from build123d import *

# Parameters (mm, degrees)
F0_R     = 19.355113
F1_DEPTH = 17.5
F2_R     = 5
F3_R     = 5


with BuildPart() as f1:
    # F0 (on Front) → F1 (new body, symmetric)
    with BuildSketch(Plane.XZ):
        Circle(F0_R)
    extrude(amount=F1_DEPTH, both=True)

    # F2
    f2_edges = [f1.edges().sort_by_distance(p)[0] for p in [
        (-19.355113, -17.5, 0),
    ]]
    fillet(f2_edges, radius=F2_R)

    # F3
    f3_edges = [f1.edges().sort_by_distance(p)[0] for p in [
        (-19.355113, 17.5, 0),
    ]]
    fillet(f3_edges, radius=F3_R)


solid = f1.part
The listing builds one solid part. Answer for the finished solid, in the listing's coordinates (mm). Round coordinates to 2 decimals unless told otherwise and drop trailing zeros. Write each loop counter-clockwise with the first axis right and the second up, starting at its lowest first coordinate (ties: lowest second). Pieces come first, ordered by that corner, then holes. Notation, with made-up numbers: M 2.5,84.25 L 32.5,84.25 A11 ccw 32.5,101.25 Z; hole C -29,-11.75 d2. An arc over 180 degrees is marked long. Write each question's results on one line, items separated by ' | '. Start each with the question number.
Item 1: Flat-ended cylindrical pins translate along their axes: pin 1 Ø1.5 at (x, z) = (13.5, 13.5) entering from +Y; pin 2 Ø6 at (x, y) = (-11, 7) entering from +Z; pin 3 Ø5 at (x, y) = (10, -7) entering from +Z. Find the tip coordinate at first contact, or state that the pin passes through.
Item 2: For a pull along X with two mould halves and no side action, classify faces 1 (the face through (0, -17.5, 0)), 2 (the face through (18.461, -0.175, 5.814)) as pulls with the +X half, pulls with the -X half, needs draft (parallel to the pull), parting line crosses it, or undercut.
Item 3: A cutting plane is placed at C-C on y = 10.5. Write down the section's boundary in (x, z), and give its area (3 significant figures).
Item 4: A cutting plane is placed at B-B on z = 0. Write down the section's boundary in (x, y), and give its area (3 significant figures).
Item 5: A cutting plane is placed at A-A on x = 0. Write down the section's boundary in (y, z).
Item 6: Straight lines are drawn through the part: L1, parallel to Y at x = -11.5, z = 12.5; L2, parallel to Y at x = 14, z = -5; L3, parallel to X at y = -5, z = 11. For each, find the intervals that lie inside material, in ascending order. Write a range as [from, to].
Check sheet entries:
1) pin 1: y = 15.52 | pin 2: z = 17.62 | pin 3: z = 17.84
2) face 1: needs draft | face 2: parting line crosses it
3) outline: C 0,0 d38.71 | area: 1,180 mm²
4) outline: M -19.36,-12.5 A5 ccw -14.36,-17.5 L 14.36,-17.5 A5 ccw 19.36,-12.5 L 19.36,12.5 A5 ccw 14.36,17.5 L -14.36,17.5 A5 ccw -19.36,12.5 Z | area: 1,330 mm²
5) outline: M -17.5,-14.36 A5 ccw -12.5,-19.36 L 12.5,-19.36 A5 ccw 17.5,-14.36 L 17.5,14.36 A5 ccw 12.5,19.36 L -12.5,19.36 A5 ccw -17.5,14.36 Z
6) L1: [-16.75, 16.75] | L2: [-17.47, 17.47] | L3: [-15.93, 15.93]
